from build123d import *

# Parameters (mm, degrees)
F0_R     = 5
F1_DEPTH = 25
F2_SIZE  = 1


with BuildPart() as f1:
    # F0 (on Right) → F1 (new body)
    with BuildSketch(Plane.YZ):
        Polygon((4.75, 8.227241), (-4.75, 8.227241), (-9.5, 0), (-4.75, -8.227241), (4.75, -8.227241), (9.5, 0), align=None)
        Circle(F0_R, mode=Mode.SUBTRACT)
    extrude(amount=F1_DEPTH)

    # F2
    f2_edges = [f1.edges().sort_by_distance(p)[0] for p in [
        (0, -5, 0),
        (25, -5, 0),
    ]]
    chamfer(f2_edges, length=F2_SIZE)


solid = f1.part
Design review of the part built by this model. Coordinates are the model's own, in mm. Coordinates: 2 decimals unless noted, no trailing zeros. Write each loop counter-clockwise with the first axis right and the second up, starting at its lowest first coordinate (ties: lowest second). Pieces come first, ordered by that corner, then holes. Notation, with made-up numbers: (70, -6) - (120, -6) arc R12 cw to (120, 8) - close; hole circle Ø8 at (54.5, -19.5). An arc over 180 degrees is marked (long way). One line per item, written item: value.
1) Add section D-D (y = 7). State the section outline as (x, z) points, plus the area to 3 significant figures.
Answer sheet:
outline: (0, -4.33) - (25, -4.33) - (25, 4.33) - (0, 4.33) - close
area: 217 mm2
2) Mouldability with a two-part tool opening along Z and no side actions: class faces 1 (the face through (25, 6.2, 0.1)), 2 (the face through (12.325, 7.158, 4.056)), 3 (the face through (12.34, -1.08, -4.88)), 4 (the face through (12, 0, -8.227)) as +Z half, -Z half, draft (parallel to the pull), parting line (faces both ways), or undercut.
Answer sheet:
face 1: draft
face 2: +Z half
face 3: undercut
face 4: -Z half
3) Add section A-A (x = 16.25). State the section outline as (y, z) points, plus the area to 3 significant figures.
Answer sheet:
outline: (-9.5, 0) - (-4.75, -8.23) - (4.75, -8.23) - (9.5, 0) - (4.75, 8.23) - (-4.75, 8.23) - close; hole circle Ø10 at (0, 0)
area: 156 mm2
4) Add section C-C (z = 7.25). State the section outline as (x, y) points.
Answer sheet:
outline: (0, -5.31) - (25, -5.31) - (25, 5.31) - (0, 5.31) - close
5) Insertion check: pin 1 (3 mm diameter, centred on x = 21.5, z = 3, fed in from +Y); pin 2 (5 mm diameter, centred on x = 14, z = -5.5, fed in from +Y); pin 3 (6 mm diameter, centred on x = 6, z = 2, fed in from -Y). Each pin has a flat end and moves straight along its axis. Give the tip position at first contact, or say it passes through.
Answer sheet:
pin 1: stops at y = 8.63
pin 2: stops at y = 7.77
pin 3: stops at y = -9.5
6) Add section B-B (y = 0). State the section outline as (x, z) points, plus the area to 3 significant figures.
Answer sheet:
outline: (0, -8.23) - (25, -8.23) - (25, -6) - (24, -5) - (1, -5) - (0, -6) - close; (0, 6) - (1, 5) - (24, 5) - (25, 6) - (25, 8.23) - (0, 8.23) - close
area: 159 mm2
7) To check wall thickness, follow probe 1 along Z at (x, y) = (10.5, 0); probe 2 along Y at (x, z) = (17.25, 1.75); probe 3 along Y at (x, z) = (22.5, -2.5). State the ranges of each line that lie inside material, in increasing order.
Answer sheet:
probe 1: z = -8.23 to -5, 5 to 8.23
probe 2: y = -8.49 to -4.68, 4.68 to 8.49
probe 3: y = -8.06 to -4.33, 4.33 to 8.06
